```python
from build123d import *

# Parameters (mm, degrees)
SKETCH1_W           = 70
SKETCH1_H           = 35
BOSS_EXTRUDE1_DEPTH = 35
SKETCH2_W           = 50
SKETCH2_H           = 20
CUT_EXTRUDE1_DEPTH  = 36
CUT_EXTRUDE2_DEPTH  = 36
CUT_EXTRUDE3_DEPTH  = 35
SKETCH5_R           = 5
CUT_EXTRUDE4_DEPTH  = 35
SKETCH6_R           = 5
CUT_EXTRUDE5_DEPTH  = 35


with BuildPart() as part:
    # Sketch1 → Boss-Extrude1 (new body)
    with BuildSketch(Plane(origin=(0, 0, 0), x_dir=(1, 0, 0), z_dir=(0, 1, 0))):
        with Locations((35, 17.5)):
            Rectangle(SKETCH1_W, SKETCH1_H)
    extrude(amount=BOSS_EXTRUDE1_DEPTH)

    # Sketch2 → Cut-Extrude1 (cut, through all)
    with BuildSketch(Plane(origin=(0, 35, 0), x_dir=(1, 0, 0), z_dir=(0, 1, 0))):
        with Locations((35, 10)):
            Rectangle(SKETCH2_W, SKETCH2_H)
    extrude(amount=-CUT_EXTRUDE1_DEPTH, mode=Mode.SUBTRACT)

    # Sketch3 → Cut-Extrude2 (cut, through all)
    with BuildSketch(Plane(origin=(0, 0, -35), x_dir=(-1, 0, 0), z_dir=(0, 0, -1))):
        Polygon((-70, 35), (-70, 15), (-30, 35), align=None)
    extrude(amount=-CUT_EXTRUDE2_DEPTH, mode=Mode.SUBTRACT)

    # Sketch4 → Cut-Extrude3 (cut)
    with BuildSketch(Plane.ZY):
        Polygon((0, 35), (-10, 35), (0, 25), align=None)
    extrude(amount=-CUT_EXTRUDE3_DEPTH, mode=Mode.SUBTRACT)

    # Sketch5 → Cut-Extrude4 (cut)
    with BuildSketch(Plane.XY.offset(-20)):
        with Locations((20, 20)):
            Circle(SKETCH5_R)
    extrude(amount=-CUT_EXTRUDE4_DEPTH, mode=Mode.SUBTRACT)

    # Sketch6 → Cut-Extrude5 (cut)
    with BuildSketch(Plane.XY.offset(-20)):
        with Locations((45, 10)):
            Circle(SKETCH6_R)
    extrude(amount=-CUT_EXTRUDE5_DEPTH, mode=Mode.SUBTRACT)


solid = part.part
```
Verification items for the finished model (mm, model axes). A direction names the side the tool comes from. Give positions to 0.01 mm unless a question says otherwise; leave off trailing zeros. Order: outer loops, then holes, each group sorted by start corner. A loop starts at its lowest first (then second) coordinate and runs counter-clockwise, first axis right, second up. Notation, with made-up numbers: M 5.5,21.25 L 64.5,21.25 A14 cw 64.5,47.25 Z; hole C 61.25,-33.5 d1. An arc over 180 degrees is marked long. Answer in a Markdown table with one row per item. Add a question column.
Item 1: Section check C-C, the plane z = -29. Enter the section's corners in (x, y), and give its area (3 significant figures).
Item 2: Scan lines: probe 1 along Y at (x, z) = (20, -24); probe 2 along X at (y, z) = (3, -3.5); probe 3 along Z at (x, y) = (13.5, 9). Record each from-to range of solid material in increasing order. Write a range as from..to.
Item 3: Mould release check, pull along Y, two halves, no side actions. Record for faces 3 (the flat face through (54.72, 22.64, -25.52)), 4 (the flat face through (10, 18, -10)), 5 (the cylindrical face through (40, 10, -27)): released by +Y, released by -Y, zero draft, split by the parting line, or undercut.
Item 4: Tool access check on faces 1 (the flat face through (35, 18, -20)), 2 (the flat face through (27, 13, -35)). Record the directions out of +Z, -Z, +X, -X, +Y, -Y that give a thin tool (end or side, any length) a straight path to the whole face; none if there is none.
Item 5: Gauge pin test, flat ends, axial feed: pin 1 (10 mm diameter, centred on y = 17.5, z = -13.5, fed in from +X); pin 2 (1.5 mm diameter, centred on x = 59.5, z = -21, fed in from +Y) (3 decimals); pin 3 (17.5 mm diameter, centred on x = 39, y = 24, fed in from +Z). Record the tip position at first contact, or that the pin passes through.
Item 6: Section check D-D, the plane y = 29. Enter the section's corners in (x, z).
Item 7: Section check A-A, the plane z = -3. Enter the section's corners in (x, y).
Item 8: Section check B-B, the plane x = 20. Enter the section's corners in (y, z).
Filled sheet:
| question | item | result |
|---|---|---|
| 1 | outline | M 0,0 L 70,0 L 70,15 L 30,35 L 0,35 Z; hole C 20,20 d10; hole C 45,10 d10 |
| 1 | area | 1,890 mm^2 |
| 2 | probe 1 | y = 0..15, 25..35 |
| 2 | probe 2 | x = 0..10, 60..70 |
| 2 | probe 3 | z = -35..-20 |
| 3 | face 3 | released by +Y |
| 3 | face 4 | zero draft |
| 3 | face 5 | undercut |
| 4 | face 1 | +Z, +Y, -Y |
| 4 | face 2 | -Z, +X, -X, +Y, -Y |
| 5 | pin 1 | stops at x = 70 |
| 5 | pin 2 | stops at y = 20.625 |
| 5 | pin 3 | stops at z = -20 |
| 6 | outline | M 0,-35 L 42,-35 L 42,-20 L 10,-20 L 10,-4 L 0,-4 Z |
| 7 | outline | M 0,0 L 10,0 L 10,28 L 0,28 Z; M 60,0 L 70,0 L 70,15 L 60,20 Z |
| 8 | outline | M 0,-35 L 15,-35 L 15,-20 L 0,-20 Z; M 25,-35 L 35,-35 L 35,-20 L 25,-20 Z |
